```python
from build123d import *

# Parameters (mm, degrees)
BOSS_EXTRUDE1_DEPTH = 48.26
SKETCH4_W           = 41.656
SKETCH4_H           = 22.86
CUT_EXTRUDE1_DEPTH  = 25.4
CUT_EXTRUDE2_DEPTH  = 25.4
SKETCH6_W           = 43.18
SKETCH6_H           = 2.54
BOSS_EXTRUDE2_DEPTH = 0.508
CHAMFER2_SIZE       = 3.048
CHAMFER3_SIZE       = 3.81


with BuildPart() as part:
    # Sketch1 → Boss-Extrude1 (new body)
    with BuildSketch(Plane.XY):
        with BuildLine():
            Line((0, 0), (0, 2.54))
            ThreePointArc((0, 2.54), (30.099, -1.078274453), (60.198, 2.54))
            Line((60.198, 2.54), (60.198, 0))
            ThreePointArc((60.198, 0), (30.099, -3.618274453), (0, 0))
        make_face()
    extrude(amount=BOSS_EXTRUDE1_DEPTH)

    # Sketch4 → Cut-Extrude1 (cut)
    with BuildSketch(Plane(origin=(0, 3.81, 0), x_dir=(1, 0, 0), z_dir=(0, 1, 0))):
        with Locations((39.37, -24.13)):
            Rectangle(SKETCH4_W, SKETCH4_H)
    extrude(amount=-CUT_EXTRUDE1_DEPTH, mode=Mode.SUBTRACT)

    # Sketch5 → Cut-Extrude2 (cut)
    with BuildSketch(Plane(origin=(0, 3.81, 0), x_dir=(1, 0, 0), z_dir=(0, 1, 0))):
        Polygon((33.782, -12.7), (33.782, -5.08), (56.388, -5.08), (56.388, -2.54), (60.198, -2.54), (60.198, -3.81), (60.198, -12.7), align=None)
        Polygon((33.782, -35.56), (60.198, -35.56), (60.198, -45.72), (56.388, -45.72), (56.388, -43.18), (33.782, -43.18), align=None)
    extrude(amount=-CUT_EXTRUDE2_DEPTH, mode=Mode.SUBTRACT)

    # Sketch6 → Boss-Extrude2 (add)
    with BuildSketch(Plane.ZY):
        with Locations((24.13, 1.27)):
            Rectangle(SKETCH6_W, SKETCH6_H)
    extrude(amount=BOSS_EXTRUDE2_DEPTH)

    # Chamfer2
    # the kernel refuses this chamfer: 3.048 mm, written as the material it takes off along each edge
    with BuildSketch(Plane(origin=(56.388, 9.510915582, 43.18), x_dir=(0.02749587661058498, 0, 0.9996219169112968), z_dir=(0, -1, 0))) as chamfer2_piece_1_section:
        Polygon((CHAMFER2_SIZE * 0.999621916911, CHAMFER2_SIZE * 0.0274958766106), (-CHAMFER2_SIZE * 0.0274958766106, CHAMFER2_SIZE * 0.999621916911), (0, 0), align=None)
    chamfer2_piece_1 = extrude(amount=18.216979495, mode=Mode.PRIVATE)
    chamfer2_piece_1 = split(chamfer2_piece_1, bisect_by=Plane(origin=(55.345503153, 0.402425835, 45.72), z_dir=(0, 0, -1)), keep=Keep.TOP, mode=Mode.PRIVATE)
    add(chamfer2_piece_1, mode=Mode.SUBTRACT)
    with BuildSketch(Plane(origin=(56.388, 9.510915582, 5.08), x_dir=(-0.9996219169112968, 0, 0.027495876610586396), z_dir=(0, -1, 0))) as chamfer2_piece_2_section:
        Polygon((CHAMFER2_SIZE * 0.999621916911, CHAMFER2_SIZE * 0.0274958766106), (-CHAMFER2_SIZE * 0.0274958766106, CHAMFER2_SIZE * 0.999621916911), (0, 0), align=None)
    chamfer2_piece_2 = extrude(amount=18.216979495, mode=Mode.PRIVATE)
    chamfer2_piece_2 = split(chamfer2_piece_2, bisect_by=Plane(origin=(55.345503153, 0.402425835, 2.54), z_dir=(0, 0, 1)), keep=Keep.TOP, mode=Mode.PRIVATE)
    add(chamfer2_piece_2, mode=Mode.SUBTRACT)

    # Chamfer3
    chamfer3_edges = [part.edges().sort_by_distance(p)[0] for p in [
        (33.782, -2.29485972, 12.7),
        (33.782, -2.29485972, 35.56),
    ]]
    chamfer(chamfer3_edges, length=CHAMFER3_SIZE)


solid = part.part
```
Part model, mm, in its own coordinate system. A direction names the side the tool comes from. Round coordinates to 2 decimals unless told otherwise and drop trailing zeros. Loops run counter-clockwise (first coordinate to the right, second up) from the corner with the lowest first, then second, coordinate; pieces in that order, holes last. Notation, with made-up numbers: (-9, -6.5) -> (14, -6.5) arc R18 cw to (14, 7.5) -> close; hole circle Ø9 at (7, 56.5). An arc over 180 degrees is marked (long way). Use one line per item in the form item = value. Start each with the question number.
Item 1: Two-plate mould, pull along Z, no slides. Class faces 1 (the flat face through (24, -2, 35.56)), 2 (the flat face through (54.63, 0.07, 44.47)), 3 (the flat face through (60.198, 1, 47)), 4 (the flat face through (31, -2, 0)): released by +Z, released by -Z, zero draft, split by the parting line, or undercut.
Item 2: Tool access for faces 5 (the flat face through (0, 1, 1)), 6 (the flat face through (0, 1, 47)), 7 (the flat face through (60.198, 1, 1)), 8 (the flat face through (18.542, -2, 24)), 9 (the cylindrical face through (17.042, -2.945, 23.792)): list every direction of +Z, -Z, +X, -X, +Y, -Y with a clear straight run to the whole face (end or side of a thin tool).
Item 3: Band-saw the part on C-C (z = 37). List the corners of the cut face in (x, y), plus the area to 3 significant figures.
Item 4: Drop flat-ended pins along their axis: pin 1 Ø10 at (x, z) = (43, 40) entering from +Y; pin 2 Ø2.5 at (x, y) = (26, -1.5) entering from -Z; pin 3 Ø1.3 at (y, z) = (-2, 18.5) entering from +X; pin 4 Ø2 at (y, z) = (1.5, 47) entering from -X. Give the stop position or say it passes through.
Item 5: Band-saw the part on B-B (z = 20). List the corners of the cut face in (x, y).
Item 6: Band-saw the part on D-D (x = 6.5). List the corners of the cut face in (y, z), plus the area to 3 significant figures.
Item 7: Drill centre lines: line 1 along Z through (x, y) = (43, -0.5); line 2 along Z through (x, y) = (19, -1); line 3 along Y through (x, z) = (11.5, 44.5). Where is each one in solid material? Low to high.
Item 8: Band-saw the part on A-A (x = 37). List the corners of the cut face in (y, z).
Data:
q1.face_1 = undercut
q1.face_2 = undercut
q1.face_3 = zero draft
q1.face_4 = released by -Z
q2.face_5 = -Z, -X, +Y, -Y
q2.face_6 = +Z, -X, +Y, -Y
q2.face_7 = +Z, -Z, +X, +Y, -Y
q2.face_8 = +X, +Y, -Y
q2.face_9 = +Z, -Z, -Y
q3.outline = (-0.51, 0) -> (0, 0) arc R127 ccw to (31.41, -3.61) -> (31.41, -1.07) arc R127 cw to (0, 2.54) -> (-0.51, 2.54) -> close
q3.area = 81.1 mm^2
q4.pin_1 = 0.03
q4.pin_2 = 0
q4.pin_3 = 18.54
q4.pin_4 = 0
q5.outline = (-0.51, 0) -> (0, 0) arc R127 ccw to (18.54, -3.09) -> (18.54, -0.55) arc R127 cw to (0, 2.54) -> (-0.51, 2.54) -> close
q6.outline = (-1.41, 0) -> (1.13, 0) -> (1.13, 48.26) -> (-1.41, 48.26) -> close
q6.area = 123 mm^2
q7.line_1 = 0 to 5.08, 43.18 to 48.26
q7.line_2 = 0 to 12.7, 35.56 to 48.26
q7.line_3 = -2.25 to 0.29
q8.outline = (-3.43, 0) -> (-0.89, 0) -> (-0.89, 5.08) -> (-3.43, 5.08) -> close; (-3.43, 43.18) -> (-0.89, 43.18) -> (-0.89, 48.26) -> (-3.43, 48.26) -> close
